```python
from build123d import *

# Parameters (mm, degrees)
SKETCH1_W           = 177.8
SKETCH1_H           = 177.8
BOSS_EXTRUDE1_DEPTH = 50.8
SHELL1_T            = -2.54
RIB2_START          = -1.905
RIB2_DEPTH          = 3.81
RIB3_REACH          = 134.129


# Read off the part's stored shape, not the designer's step: Rib2
with BuildPart() as part:
    # Sketch1 → Boss-Extrude1 (new body)
    with BuildSketch(Plane(origin=(0, 0, 0), x_dir=(1, 0, 0), z_dir=(0, 1, 0))):
        Rectangle(SKETCH1_W, SKETCH1_H)
    extrude(amount=BOSS_EXTRUDE1_DEPTH)

    # Shell1
    shell1_openings = [part.faces().sort_by_distance(p)[0] for p in [
        (0, 50.8, 0),
    ]]
    offset(amount=SHELL1_T, openings=shell1_openings, kind=Kind.INTERSECTION)

    # Rib2 outline → Rib2 (add)
    with BuildSketch(Plane.XY.offset(RIB2_START)):
        Polygon((-48.26, 2.54), (-86.36, 40.64), (-86.36, 2.54), align=None)
    rib2 = extrude(amount=RIB2_DEPTH)

    # Mirror1: Rib2 across plane
    add(rib2.mirror(Plane(origin=(0, 0, 0), x_dir=(0, 0, 1), z_dir=(1, 0, 0))))

    # Sketch3 walls → Rib3 (add, up to next)
    with BuildSketch(Plane(origin=(0, 40.64, 0), x_dir=(1, 0, 0), z_dir=(0, 1, 0)), mode=Mode.PRIVATE) as rib3_sk1:
        with BuildLine():
            Line((1.905, -219.488837125), (1.905, -20.868229441))
            ThreePointArc((1.905, -20.868229441), (20.955, 0), (1.905, 20.868229441))
            Line((1.905, 20.868229441), (1.905, 219.488837125))
            Line((1.905, 219.488837125), (-1.905, 219.488837125))
            Line((-1.905, 219.488837125), (-1.905, 17.038837989))
            ThreePointArc((-1.905, 17.038837989), (17.145, 0), (-1.905, -17.038837989))
            Line((-1.905, -17.038837989), (-1.905, -219.488837125))
            Line((-1.905, -219.488837125), (1.905, -219.488837125))
        make_face()
    rib3_tool1 = extrude(rib3_sk1.sketch, amount=-RIB3_REACH, mode=Mode.PRIVATE) - part.part
    add(rib3_tool1.solids().sort_by_distance((19.05, 40.64, 0))[0])


solid = part.part
```
Read the model definition and answer for the solid it produces. Units are mm, in the model's axes. A direction names the side the tool comes from. Give positions to 0.01 mm unless a question says otherwise; leave off trailing zeros. Order: outer loops, then holes, each group sorted by start corner. A loop starts at its lowest first (then second) coordinate and runs counter-clockwise, first axis right, second up. Notation, with made-up numbers: (-13.75, -37.5) -> (17.25, -37.5) arc R11 cw to (17.25, -29.5) -> close; hole circle Ø7 at (33.25, -25). An arc over 180 degrees is marked (long way). One line per item, written item: value. Start each with the question number.
(1) A flat-ended cylindrical pin translates along its axis: P1, Ø18.5, axis at x = 6, z = 1.5, coming from the +Y side. Find the tip coordinate at first contact, or state that the pin passes through.
(2) The part is cut by section D-D (x = -72). Determine the outline of the cut face in (y, z) (3 decimals).
(3) Straight lines are drawn through the part: L1, parallel to Z at x = 59, y = 10 (3 decimals); L2, parallel to Z at x = 25, y = 10. For each, find the intervals that lie inside material, in ascending order.
(4) A tool of negligible diameter and unlimited length cuts with its end or side. For faces 1 (the flat face through (-86.36, 42, 1)), 2 (the flat face through (-1, 0, -1)), from which of +Z, -Z, +X, -X, +Y, -Y can it reach the whole face along a straight path? Write none if from no direction.
(5) The part is cut by section B-B (y = 44.5). Determine the outline of the cut face in (x, z).
(6) The part is cut by section A-A (y = 6). Determine the outline of the cut face in (x, z) (3 decimals).
(7) For a pull along X with two mould halves and no side action, classify faces 3 (the flat face through (-88.9, 25, 1)), 4 (the flat face through (1.905, 22, 54)), 5 (the flat face through (-1, 25, -88.9)) as released by +X, released by -X, zero draft, split by the parting line, or undercut.
(8) The part is cut by section C-C (z = 78.5). Determine the outline of the cut face in (x, y) (3 decimals).
Taken from the geometry:
1. P1: y = 2.54
2. outline: (0, -88.9) -> (50.8, -88.9) -> (50.8, -86.36) -> (2.54, -86.36) -> (2.54, -1.905) -> (26.28, -1.905) -> (26.28, 1.905) -> (2.54, 1.905) -> (2.54, 86.36) -> (50.8, 86.36) -> (50.8, 88.9) -> (0, 88.9) -> close
3. L1: -88.9 to -86.36, -1.905 to 1.905, 86.36 to 88.9
3. L2: -88.9 to -86.36, 86.36 to 88.9
4. face 1: +Y
4. face 2: +Z, -Z, +X, -X, -Y
5. outline: (-88.9, -88.9) -> (88.9, -88.9) -> (88.9, 88.9) -> (-88.9, 88.9) -> close; hole (-86.36, -86.36) -> (86.36, -86.36) -> (86.36, 86.36) -> (-86.36, 86.36) -> close
6. outline: (-88.9, -88.9) -> (88.9, -88.9) -> (88.9, 88.9) -> (-88.9, 88.9) -> close; hole (-86.36, -86.36) -> (-1.905, -86.36) -> (-1.905, -17.039) arc R17.145 ccw (long way) to (-1.905, 17.039) -> (-1.905, 86.36) -> (-86.36, 86.36) -> (-86.36, 1.905) -> (-51.72, 1.905) -> (-51.72, -1.905) -> (-86.36, -1.905) -> close; hole (1.905, -86.36) -> (86.36, -86.36) -> (86.36, -1.905) -> (51.72, -1.905) -> (51.72, 1.905) -> (86.36, 1.905) -> (86.36, 86.36) -> (1.905, 86.36) -> (1.905, 20.868) arc R20.955 cw to (1.905, -20.868) -> close
7. face 3: released by -X
7. face 4: undercut
7. face 5: zero draft
8. outline: (-88.9, 0) -> (88.9, 0) -> (88.9, 50.8) -> (86.36, 50.8) -> (86.36, 2.54) -> (1.905, 2.54) -> (1.905, 40.64) -> (-1.905, 40.64) -> (-1.905, 2.54) -> (-86.36, 2.54) -> (-86.36, 50.8) -> (-88.9, 50.8) -> close
